Drawing for the job (mm, zero at the part's lowest x, y, z). Coordinates: 2 decimals unless noted, no trailing zeros. Write each loop counter-clockwise with the first axis right and the second up, starting at its lowest first coordinate (ties: lowest second). Pieces come first, ordered by that corner, then holes. Notation, with made-up numbers: (65.25, 81) -> (117.25, 81) arc R22 cw to (117.25, 117) -> close; hole circle Ø5 at (62.25, -9.5). An arc over 180 degrees is marked (long way). Write each question's results on one line, items separated by ' | '. Start each with the question number.
Q1. Drill centre lines: line 1 (X direction, y = 126.5, z = 14.5); line 2 (Y direction, x = 727, z = 27.5). Where is each one in solid material? Low to high.
Q2. Saw through at B-B on x = 406.5. Give the cut face in (y, z).
Q3. Saw through at C-C on z = 38.5. Give the cut face in (x, y), and give its area (3 significant figures).
Q4. Saw through at A-A on y = 143. Give the cut face in (x, z), and give its area (3 significant figures).
Q5. Drop a flat-ended pin along its axis: pin 1 Ø3 at (y, z) = (599.5, 26.5) entering from -X. Give the stop position or say it passes through.
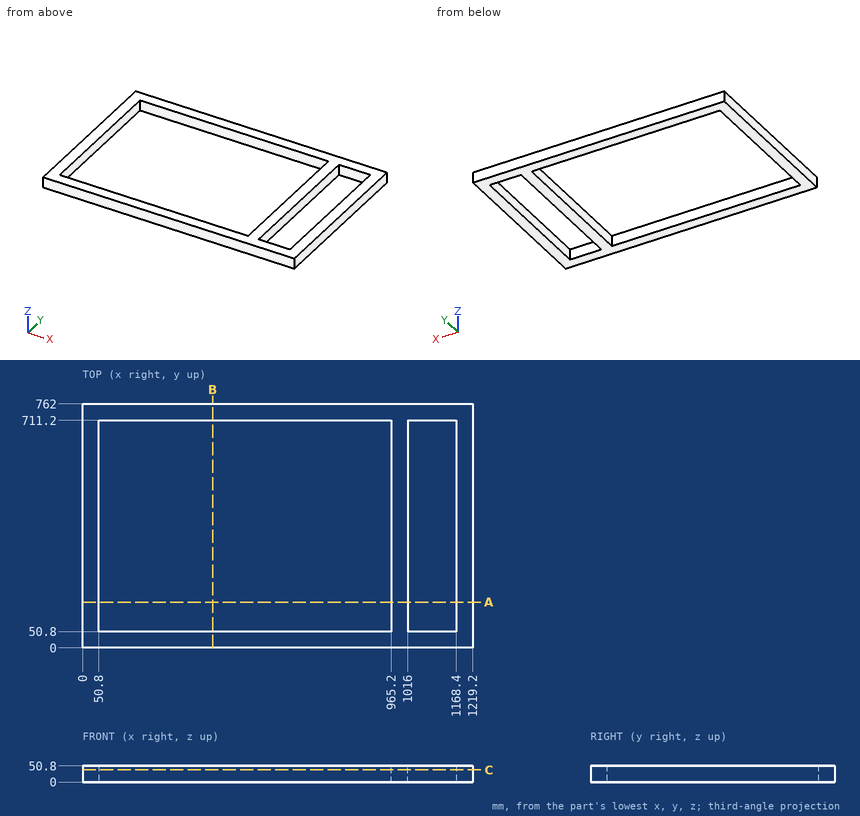
Returned:
1) line 1: x = 0 to 50.8, 965.2 to 1016, 1168.4 to 1219.2 | line 2: y = 0 to 50.8, 711.2 to 762
2) outline: (0, 0) -> (50.8, 0) -> (50.8, 50.8) -> (0, 50.8) -> close; (711.2, 0) -> (762, 0) -> (762, 50.8) -> (711.2, 50.8) -> close
3) outline: (0, 0) -> (1219.2, 0) -> (1219.2, 762) -> (0, 762) -> close; hole (50.8, 50.8) -> (965.2, 50.8) -> (965.2, 711.2) -> (50.8, 711.2) -> close; hole (1016, 50.8) -> (1168.4, 50.8) -> (1168.4, 711.2) -> (1016, 711.2) -> close | area: 225,000 mm2
4) outline: (0, 0) -> (50.8, 0) -> (50.8, 50.8) -> (0, 50.8) -> close; (965.2, 0) -> (1016, 0) -> (1016, 50.8) -> (965.2, 50.8) -> close; (1168.4, 0) -> (1219.2, 0) -> (1219.2, 50.8) -> (1168.4, 50.8) -> close | area: 7,740 mm2
5) pin 1: stops at x = 0
